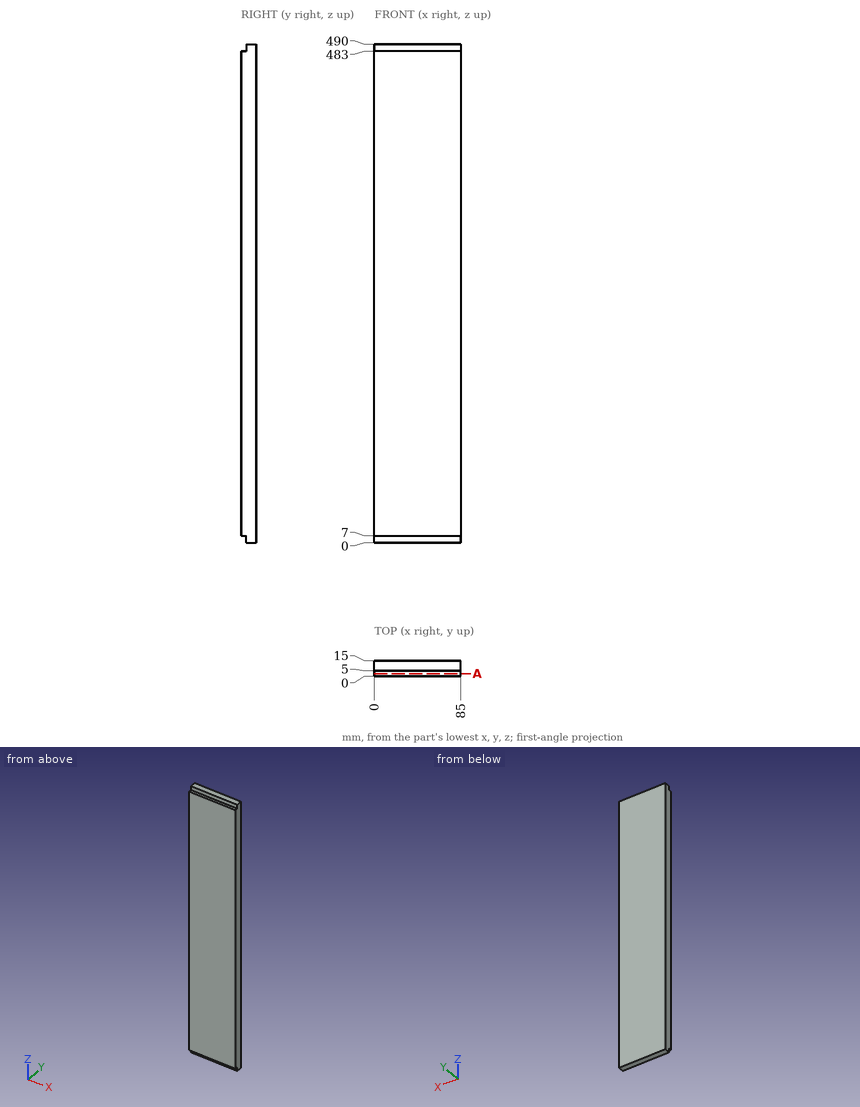
Job drawing, mm, ordinate dimensions from the low corner. One solid piece. Round coordinates to 2 decimals unless told otherwise and drop trailing zeros. Write each loop counter-clockwise with the first axis right and the second up, starting at its lowest first coordinate (ties: lowest second). Pieces come first, ordered by that corner, then holes. Notation, with made-up numbers: (35, 69.5) -> (57, 69.5) arc R22 ccw to (57, 107.5) -> close; hole circle Ø10 at (65, -21). An arc over 180 degrees is marked (long way). Answer as a JSON object with one key per item and string values.
(1) Probe probe 1 along Z at (x, y) = (57, 2.5). List the from-to ranges inside material, lowest first. Write a range as [from, to].
Reported:
{"probe 1": "z = [7, 483]"}
(2) Band-saw the part on A-A, the plane y = 2.25. List the corners of the cut face in (x, z), then the cut area to 3 significant figures.
Reported:
{"outline": "(0, 7) -> (85, 7) -> (85, 483) -> (0, 483) -> close", "area": "40,500 mm^2"}
(3) Pin check, flat tips, straight feed: P1, Ø2, axis at x = 57.5, y = 10.5, coming from the -Z side; P2, Ø3.5, axis at x = 43, z = 3.5, coming from the -Y side; P3, Ø4, axis at x = 31.5, y = 2.5, coming from the +Z side; P4, Ø4, axis at x = 48.5, y = 2.5, coming from the -Z side. Stop position of each tip, or through.
Reported:
{"P1": "stops at z = 0", "P2": "stops at y = 5", "P3": "stops at z = 483", "P4": "stops at z = 7"}
